```python
from build123d import *

# Parameters (mm, degrees)
F0_W     = 400
F0_H     = 350
F1_DEPTH = 19
F3_DEPTH = 19.001


with BuildPart() as f1:
    # F0 (on Top) → F1 (new body)
    with BuildSketch(Plane.XY):
        Rectangle(F0_W, F0_H)
    extrude(amount=F1_DEPTH)

    # F2 (on face) → F3 (cut, through all)
    with BuildSketch(Plane.XY.offset(19)):
        Polygon((-200, 175), (-200, 125.820249), (-144.6933, 175), align=None)
        Polygon((200, -125.820249), (144.693285, -175), (200, -175), align=None)
        Polygon((-137.878031, -175), (-200, -133.684024), (-200, -175), align=None)
        Polygon((200, 175), (133.159757, 175), (200, 129.490018), align=None)
    extrude(amount=-F3_DEPTH, mode=Mode.SUBTRACT)


solid = f1.part
```
CAD build for the part. Positions are in the model's coordinates, mm. Round coordinates to 2 decimals unless told otherwise and drop trailing zeros. Write each loop counter-clockwise with the first axis right and the second up, starting at its lowest first coordinate (ties: lowest second). Pieces come first, ordered by that corner, then holes. Notation, with made-up numbers: (9, -23.5) - (15, -23.5) arc R14 cw to (15, -10.5) - close; hole circle Ø8 at (48, 86.5). An arc over 180 degrees is marked (long way). Write item = value, one per line. Start each with the question number.
Q1. Drop flat-ended pins along their axis: pin 1 (1 mm diameter, centred on x = 158.5, z = 9, fed in from -Y); pin 2 (2 mm diameter, centred on x = 158, y = 116.5, fed in from -Z). Give the stop position or say it passes through.
Q2. Band-saw the part on A-A (z = 16). Give the cut face in (x, y).
Q3. Probe L1, parallel to Y at x = 145.5, z = 1.75; L2, parallel to X at y = -136.5, z = 14.75; L3, parallel to Y at x = -171.5, z = 7.5. List the from-to ranges inside material, lowest first. Write a range as from..to.
Answers below:
q1.pin_1 = -163.17
q1.pin_2 = 0
q2.outline = (-200, -133.68) - (-137.88, -175) - (144.69, -175) - (200, -125.82) - (200, 129.49) - (133.16, 175) - (-144.69, 175) - (-200, 125.82) - close
q3.L1 = -174.28..166.6
q3.L2 = -195.77..187.99
q3.L3 = -152.64..151.16
